Geometry: final body of the model. Coordinates: model frame, mm. A direction names the side the tool comes from. Coordinates: 2 decimals unless noted, no trailing zeros. Order: outer loops, then holes, each group sorted by start corner. A loop starts at its lowest first (then second) coordinate and runs counter-clockwise, first axis right, second up. Notation, with made-up numbers: M 69,1 L 128,1 A19 ccw 128,24 Z; hole C -24,71 d11. An arc over 180 degrees is marked long. Use CSV: the item, a comma, the result in double quotes. Start each with the question number.
Q1. Access query for faces 1 (the face through (0.07, -0.51, 2.05)), 2 (the face through (1.5, 1.28, -0.07)). Directions: +Z, -Z, +X, -X, +Y, -Y. A direction counts if a zero-diameter tool reaches every point of the face in a straight line with its end or side. Return the directions, or none.
Q2. Section query B-B, the plane z = 0. Output: boundary loops of the cut face in (x, y).
Q3. Section query A-A, the plane y = -1.5. Output: boundary loops of the cut face in (x, z).
Q4. First-contact query: P1, Ø0.6, axis at y = -3, z = 1, coming from the -X side; P2, Ø1.1, axis at x = 0.5, z = 0.5, coming from the +Y side. Flat tips, straight axial feed; report the tip coordinate or a pass-through.
Q5. Ray query, probe 1 along Y at (x, z) = (-1.5, -1.15); probe 2 along X at (y, z) = (2.5, -1.1); probe 3 along X at (y, z) = (-1.5, 1.45). Return the intervals inside material, ascending.
Q6. Section query D-D, the plane y = 0.5. Output: boundary loops of the cut face in (x, z).
from build123d import *

# Parameters (mm, degrees)
CUT_EXTRUDE1_DEPTH  = 2
SKETCH3_W           = 0.5
SKETCH3_H           = 0.5
BOSS_EXTRUDE1_DEPTH = 3


with BuildPart() as part:
    # Sketch1 → Revolve1 (revolve)
    with BuildSketch(Plane.XY):
        with BuildLine():
            Line((-1.5, 2.6), (-1.5, 0))
            Line((-1.5, 0), (-2.05, 0))
            Line((-2.05, 0), (-2.05, -1))
            Line((-2.05, -1), (0, -1))
            Line((0, -1), (0, 4.1))
            ThreePointArc((0, 4.1), (-1.060660172, 3.660660172), (-1.5, 2.6))
        make_face()
    revolve(axis=Axis((0, 4.1, 0), (0, -1, 0)))

    # Sketch2 → Cut-Extrude1 (cut, through all)
    with BuildSketch(Plane(origin=(0, 0, 0), x_dir=(1, 0, 0), z_dir=(0, 1, 0))):
        Polygon((-1.949403326, 1.5), (2.097394678, 1.5), (0.505211857, 3.403801095), align=None)
    extrude(amount=-CUT_EXTRUDE1_DEPTH, mode=Mode.SUBTRACT)

    # Sketch3 → Boss-Extrude1 (add)
    with BuildSketch(Plane.XZ.offset(1)):
        with Locations((0, 1.27)):
            Rectangle(SKETCH3_W, SKETCH3_H)
        with Locations((0, -1.27)):
            Rectangle(SKETCH3_W, SKETCH3_H)
    extrude(amount=BOSS_EXTRUDE1_DEPTH)


solid = part.part
Responses:
1,face 1,"+Y, -Y"
1,face 2,"+Y"
2,outline,"M -2.05,-1 L 2.05,-1 L 2.05,0 L 1.5,0 L 1.5,2.6 A1.5 ccw -1.5,2.6 L -1.5,0 L -2.05,0 Z"
3,outline,"M -0.25,-1.52 L 0.25,-1.52 L 0.25,-1.02 L -0.25,-1.02 Z; M -0.25,1.02 L 0.25,1.02 L 0.25,1.52 L -0.25,1.52 Z"
4,P1,"stops at x = -0.25"
4,P2,"stops at y = 4.09"
5,probe 1,"y = -1 to 0"
5,probe 2,"x = -1.02 to 1.02"
5,probe 3,"x = -0.25 to 0.25"
6,outline,"C 0,0 d3"
